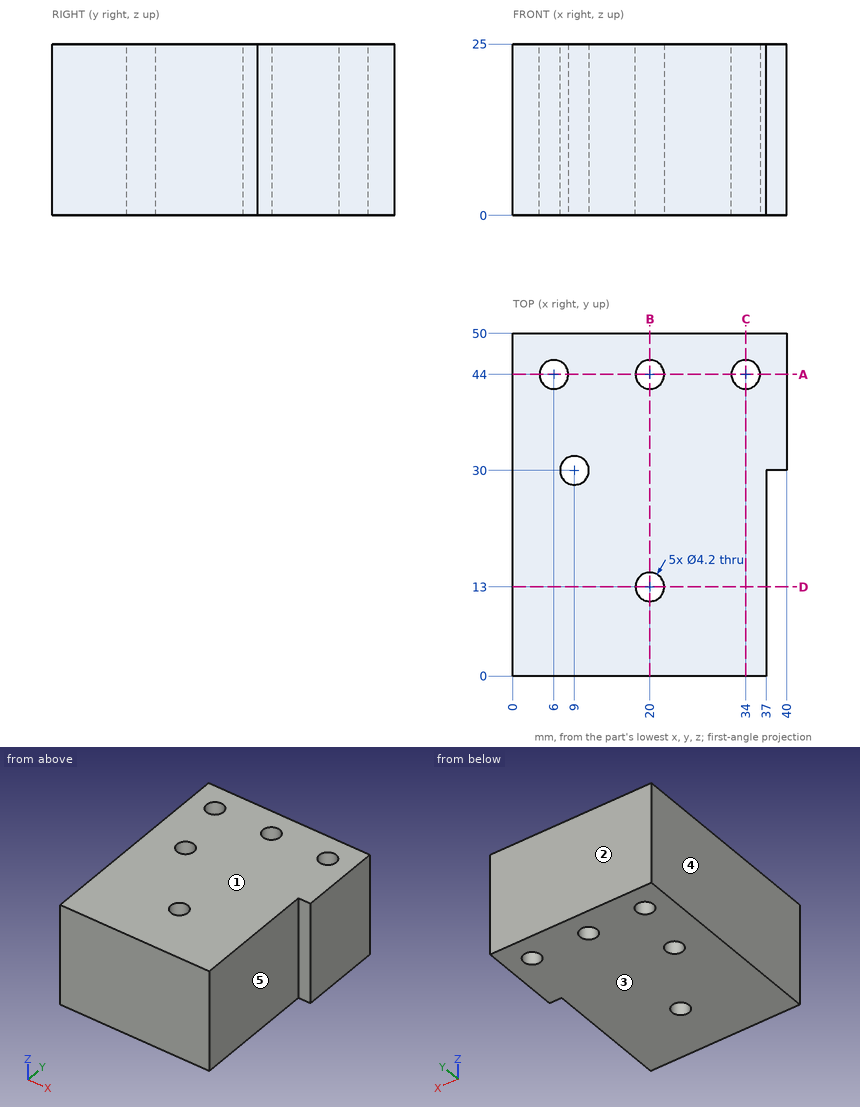
The drawing under review shows one solid part. Ordinate dimensions are in mm from its lowest x, y, z. A direction names the side the tool comes from. Coordinates: 2 decimals unless noted, no trailing zeros. Order: outer loops, then holes, each group sorted by start corner. A loop starts at its lowest first (then second) coordinate and runs counter-clockwise, first axis right, second up. Notation, with made-up numbers: (56, 20) -> (96, 20) arc R21 cw to (96, 59) -> close; hole circle Ø8 at (-19, -15). An arc over 180 degrees is marked (long way). Return JSON: item names as keys, results as strings.
1. For pin 1 Ø4 at (x, y) = (20, 44) entering from +Z, flat-tipped, find the tip position at first contact; note if it passes through.
Answer block:
{"pin 1": "through"}
2. We need section D-D on y = 13. Write out the cut boundary in (x, z).
Answer block:
{"outline": "(0, 0) -> (17.9, 0) -> (17.9, 25) -> (0, 25) -> close; (22.1, 0) -> (37, 0) -> (37, 25) -> (22.1, 25) -> close"}
3. Machinability: for the marked faces 4 and 5, which of the approach directions +Z, -Z, +X, -X, +Y, -Y give a long, thin tool a straight path to every point of the face, cutting with its end or side? Answer none if there is none.
Answer block:
{"face 4": "+Z, -Z, -X, +Y, -Y", "face 5": "+Z, -Z, +X, -Y"}
4. For line 1 (Y direction, x = 20, z = 17); line 2 (X direction, y = 9, z = 22.75); line 3 (X direction, y = 43.5, z = 12.25), list the stretches that pass through material, from the lowest coordinate up. Write a range as from..to.
Answer block:
{"line 1": "0..10.9, 15.1..41.9, 46.1..50", "line 2": "0..37", "line 3": "0..3.96, 8.04..17.96, 22.04..31.96, 36.04..40"}
5. We need section B-B on x = 20. Write out the cut boundary in (y, z), and give its area (3 significant figures).
Answer block:
{"outline": "(0, 0) -> (10.9, 0) -> (10.9, 25) -> (0, 25) -> close; (15.1, 0) -> (41.9, 0) -> (41.9, 25) -> (15.1, 25) -> close; (46.1, 0) -> (50, 0) -> (50, 25) -> (46.1, 25) -> close", "area": "1,040 mm²"}
6. The part is to be moulded in two halves that separate along Z. For the marked faces 1, 2 and 3, say which applies: +Z half, -Z half, draft (parallel to the pull), parting line (faces both ways), or undercut.
Answer block:
{"face 1": "+Z half", "face 2": "draft", "face 3": "-Z half"}
7. We need section C-C on x = 34. Write out the cut boundary in (y, z).
Answer block:
{"outline": "(0, 0) -> (41.9, 0) -> (41.9, 25) -> (0, 25) -> close; (46.1, 0) -> (50, 0) -> (50, 25) -> (46.1, 25) -> close"}
8. We need section A-A on y = 44. Write out the cut boundary in (x, z).
Answer block:
{"outline": "(0, 0) -> (3.9, 0) -> (3.9, 25) -> (0, 25) -> close; (8.1, 0) -> (17.9, 0) -> (17.9, 25) -> (8.1, 25) -> close; (22.1, 0) -> (31.9, 0) -> (31.9, 25) -> (22.1, 25) -> close; (36.1, 0) -> (40, 0) -> (40, 25) -> (36.1, 25) -> close"}
